Design review of the part built by this model. Coordinates are the model's own, in mm. Round coordinates to 2 decimals unless told otherwise and drop trailing zeros. Loops run counter-clockwise (first coordinate to the right, second up) from the corner with the lowest first, then second, coordinate; pieces in that order, holes last. Notation, with made-up numbers: (2.5, 5) -> (24.5, 5) arc R31 ccw to (24.5, 35) -> close; hole circle Ø3 at (77.5, 49.5). An arc over 180 degrees is marked (long way). Answer as CSV lines item,"result". Start each with the question number.
Autodesk Inventor part; units mm, degrees
ref_plane "YZ Plane" through (0, 0, 0) normal (1, 0, 0) x (0, 1, 0)
ref_plane "XZ Plane" through (0, 0, 0) normal (0, 1, 0) x (-1, 0, 0)
ref_plane "XY Plane" through (0, 0, 0) normal (0, 0, 1) x (1, 0, 0)
sketch "Sketch1" plane through (0, 0, 0) normal (0, 0, 1) x (1, 0, 0)
  line L0 (-40, 100) -> (40, 100)
  line L1 (40, 100) -> (40, -100)
  line L2 (40, -100) -> (-40, -100)
  line L3 (-40, -100) -> (-40, 100)
  line L4 (-40, 100) -> (40, -100) construction
  line L5 (40, 100) -> (-40, -100) construction
  point P0 (0, 0)
  dimension "d0" = 80
  dimension "d1" = 200
extrude "Extrusion1" add sketch "Sketch1" along normal blind 3
sketch "Sketch2" plane through (0, 0, 0) normal (0, 0, -1) x (-1, 0, 0)
  line L0 (40, -100) -> (-40, -100)
  line L1 (40, 100) -> (40, -100)
  line L2 (-40, 100) -> (40, 100)
  line L3 (-40, -100) -> (-40, 100)
  point P0 (0, 0)
  point P1 (32.5, -60)
  point P2 (32.5, 60)
  dimension "d4" = 7.5
  dimension "d5" = 7.5
  dimension "d6" = 40
  dimension "d7" = 40
hole "Hole1" at (-32.5, -60, 0) at (-32.5, 60, 0) direction (0, 0, 1) diameter 3.5 end through all
fillet "Fillet1" radius 3 4 edges at (-40, -100, 1.5) (40, -100, 1.5) (40, 100, 1.5) (-40, 100, 1.5)
sketch "Sketch3" plane through (0, 0, 0) normal (0, 0, -1) x (-1, 0, 0)
  arc A0 (40, 97) -> (37, 100) centre (37, 97) ccw
  line L0 (-37, 100) -> (37, 100)
  arc A1 (-37, 100) -> (-40, 97) centre (-37, 97) ccw
  line L1 (-40, -97) -> (-40, 97)
  arc A2 (-40, -97) -> (-37, -100) centre (-37, -97) ccw
  line L2 (37, -100) -> (-37, -100)
  arc A3 (37, -100) -> (40, -97) centre (37, -97) ccw
  line L3 (40, 97) -> (40, -97)
  circle A4 centre (32.5, -60) radius 1.75
  circle A5 centre (32.5, 60) radius 1.75
  line L4 (0, -85) -> (25, -85)
  line L5 (25, -85) -> (25, -38.3333)
  line L6 (25, -38.3333) -> (0, -38.3333)
  line L7 (0, -38.3333) -> (0, -85)
  line L8 (25, 85) -> (0, 85)
  line L9 (0, 85) -> (0, 38.3333)
  line L10 (0, 38.3333) -> (25, 38.3333)
  line L11 (25, 38.3333) -> (25, 85)
  line L12 (25, -23.3333) -> (0, -23.3333)
  line L13 (0, -23.3333) -> (0, 23.3333)
  line L14 (0, 23.3333) -> (25, 23.3333)
  line L15 (25, 23.3333) -> (25, -23.3333)
  point P0 (0, 0)
  point P1 (12.5, -23.3333)
  dimension "d16" = 15
  dimension "d17" = 15
  dimension "d18" = 15
  dimension "d19" = 15
  dimension "d20" = 15
  dimension "d21" = 25
extrude "Extrusion2" cut sketch "Sketch3" against normal through all contours L7 L6 L5 L4 | L11 L10 L9 L8 | L12 L13 L14 L15
equation "\"d17\" = d16"
equation "\"d18\" = d16"
equation "\"d19\" = d16"
properties part number "Drag Chain Guide Z Axis" material "Aluminum 6061"
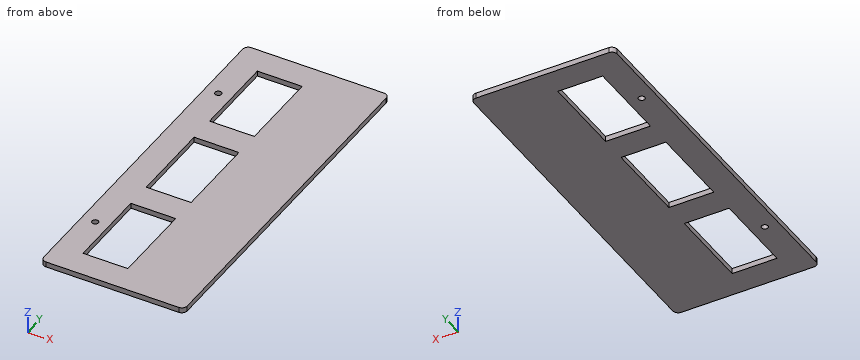
Q1. Add section B-B, the plane x = -32.5. Give the boundary of the cut face in (y, z).
Q2. To check wall thickness, follow probe 1 along X at (y, z) = (60, 2.1); probe 2 along Y at (x, z) = (-32.5, 1.15); probe 3 along Y at (x, z) = (-0.5, 2.05). State the ranges of each line that lie inside material, in increasing order. Write a range as from..to.
Q3. Add section D-D, the plane y = -7. Give the boundary of the cut face in (x, z), and give its area (3 significant figures).
Q4. Add section A-A, the plane x = -17.5. Give the boundary of the cut face in (y, z), and give its area (3 significant figures).
Q5. Add section C-C, the plane y = -60. Give the boundary of the cut face in (x, z).
Worked answers:
1,outline,"(-100, 0) -> (-61.75, 0) -> (-61.75, 3) -> (-100, 3) -> close; (-58.25, 0) -> (58.25, 0) -> (58.25, 3) -> (-58.25, 3) -> close; (61.75, 0) -> (100, 0) -> (100, 3) -> (61.75, 3) -> close"
2,probe 1,"x = -40..-34.25, -30.75..-25, 0..40"
2,probe 2,"y = -100..-61.75, -58.25..58.25, 61.75..100"
2,probe 3,"y = -100..-85, -38.33..-23.33, 23.33..38.33, 85..100"
3,outline,"(-40, 0) -> (-25, 0) -> (-25, 3) -> (-40, 3) -> close; (0, 0) -> (40, 0) -> (40, 3) -> (0, 3) -> close"
3,area,"165 mm^2"
4,outline,"(-100, 0) -> (-85, 0) -> (-85, 3) -> (-100, 3) -> close; (-38.33, 0) -> (-23.33, 0) -> (-23.33, 3) -> (-38.33, 3) -> close; (23.33, 0) -> (38.33, 0) -> (38.33, 3) -> (23.33, 3) -> close; (85, 0) -> (100, 0) -> (100, 3) -> (85, 3) -> close"
4,area,"180 mm^2"
5,outline,"(-40, 0) -> (-34.25, 0) -> (-34.25, 3) -> (-40, 3) -> close; (-30.75, 0) -> (-25, 0) -> (-25, 3) -> (-30.75, 3) -> close; (0, 0) -> (40, 0) -> (40, 3) -> (0, 3) -> close"
